```python
from build123d import *

# Parameters (mm, degrees)
SKETCH_R        = 2.25
SKETCH_R_2      = 11.25
SKETCH_R_3      = 1.75
PAD_DEPTH       = 23
POCKET_DEPTH    = 19
SKETCH003_R     = 4.05
POCKET002_DEPTH = 12


with BuildPart() as part:
    # Sketch → Pad (new body)
    with BuildSketch(Plane.XY):
        Polygon((0, 0), (105, 0), (105, 62), (20, 62), (20, 42), (0, 42), align=None)
        with Locations((35, 10)):
            Circle(SKETCH_R, mode=Mode.SUBTRACT)
        with Locations((30, 35)):
            Circle(SKETCH_R, mode=Mode.SUBTRACT)
        with Locations((84, 21)):
            Circle(SKETCH_R_2, mode=Mode.SUBTRACT)
        with Locations((68.5, 36.5)):
            Circle(SKETCH_R_3, mode=Mode.SUBTRACT)
        with Locations((99.5, 36.5)):
            Circle(SKETCH_R_3, mode=Mode.SUBTRACT)
        with Locations((68.5, 5.5)):
            Circle(SKETCH_R_3, mode=Mode.SUBTRACT)
        with Locations((99.5, 5.5)):
            Circle(SKETCH_R_3, mode=Mode.SUBTRACT)
        with Locations((10, 30)):
            Circle(SKETCH_R, mode=Mode.SUBTRACT)
        with Locations((10, 15)):
            Circle(SKETCH_R, mode=Mode.SUBTRACT)
        with Locations((39, 52)):
            Circle(SKETCH_R, mode=Mode.SUBTRACT)
        with Locations((94, 52)):
            Circle(SKETCH_R, mode=Mode.SUBTRACT)
        with Locations((55, 5)):
            Circle(SKETCH_R, mode=Mode.SUBTRACT)
        with BuildLine():
            Line((58.75, 25), (58.75, 40))
            ThreePointArc((58.75, 40), (56.5, 42.25), (54.25, 40))
            Line((54.25, 25), (54.25, 40))
            ThreePointArc((54.25, 25), (56.5, 22.75), (58.75, 25))
        make_face(mode=Mode.SUBTRACT)
    extrude(amount=PAD_DEPTH)

    # Sketch001 → Pocket (cut)
    with BuildSketch(Plane.XY.offset(23)):
        with BuildLine():
            ThreePointArc((38.485281, 42), (36.015595, 44.209377), (32.999996, 45.583006))
            Line((32.999996, 67), (32.999996, 45.583006))
            Line((20, 67), (32.999996, 67))
            Line((20, -1), (20, 67))
            Line((20, -1), (48.252269, -1))
            Line((48.252269, 11), (48.252269, -1))
            Line((48.252269, 11), (70.252269, 11))
            ThreePointArc((70.252269, 11), (71.759618, 9.202833), (73.499996, 7.630258))
            Line((73.499996, 7.630258), (73.499996, -1))
            Line((73.499996, -1), (93.499996, -1))
            Line((93.499996, -1), (93.499996, 6.902128))
            ThreePointArc((93.499996, 6.902128), (95.574295, 8.548671), (97.367695, 10.497399))
            Line((105.499996, 10.497399), (97.367695, 10.497399))
            Line((105.499996, 30.497399), (105.499996, 10.497399))
            Line((98.099621, 30.497399), (105.499996, 30.497399))
            ThreePointArc((98.099621, 30.497399), (91.98574, 36.007594), (83.999996, 38))
            Line((83.999996, 38), (83.999996, 67))
            Line((83.999996, 67), (43.999996, 67))
            Line((43.999996, 67), (43.999996, 42))
            Line((38.485281, 42), (43.999996, 42))
        make_face()
    extrude(amount=-POCKET_DEPTH, mode=Mode.SUBTRACT)

    # Sketch003 → Pocket002 (cut)
    with BuildSketch(Plane.XZ):
        with Locations((10, 16)):
            Circle(SKETCH003_R)
    extrude(amount=-POCKET002_DEPTH, mode=Mode.SUBTRACT)


solid = part.part
```
Geometry check sheet. Reference: the model listing, model coordinates, mm. A direction names the side the tool comes from. Give positions to 0.01 mm unless a question says otherwise; leave off trailing zeros. Write each loop counter-clockwise with the first axis right and the second up, starting at its lowest first coordinate (ties: lowest second). Pieces come first, ordered by that corner, then holes. Notation, with made-up numbers: (18.25, 35) -> (57.25, 35) arc R19 cw to (57.25, 45) -> close; hole circle Ø1 at (77, 23.5). An arc over 180 degrees is marked (long way). Use one line per item in the form item = value.
Item 1: Scan lines: line 1 (Y direction, x = 99.5, z = 12.5); line 2 (Y direction, x = 10, z = 13.25); line 3 (X direction, y = 32, z = 9). Record each from-to range of solid material in increasing order.
Results list:
line_1 = 0 to 3.75, 7.25 to 10.5, 30.5 to 34.75, 38.25 to 62
line_2 = 12 to 12.75, 17.25 to 27.75, 32.25 to 42
line_3 = 0 to 8.97, 11.03 to 20, 96.96 to 105
Item 2: Sectioned sample at C-C on y = 16. Enter the section's corners in (x, z).
Results list:
outline = (0, 0) -> (7.98, 0) -> (7.98, 23) -> (0, 23) -> close; (12.02, 0) -> (73.92, 0) -> (73.92, 4) -> (20, 4) -> (20, 23) -> (12.02, 23) -> close; (94.08, 0) -> (105, 0) -> (105, 4) -> (94.08, 4) -> close
Item 3: Mould release check, pull along Y, two halves, no side actions. Record for faces 1 (the flat face through (72.5, 62, 3.7)), 2 (the flat face through (93.5, 3, 14)), 3 (the cylindrical face through (99.12, 34.79, 11.34)): released by +Y, released by -Y, zero draft, split by the parting line, or undercut.
Results list:
face_1 = released by +Y
face_2 = zero draft
face_3 = undercut
Item 4: Sectioned sample at B-B on x = 99.5. Enter the section's corners in (y, z), plus the area to 3 significant figures.
Results list:
outline = (0, 0) -> (3.75, 0) -> (3.75, 23) -> (0, 23) -> close; (7.25, 0) -> (34.75, 0) -> (34.75, 23) -> (30.5, 23) -> (30.5, 4) -> (10.5, 4) -> (10.5, 23) -> (7.25, 23) -> close; (38.25, 0) -> (62, 0) -> (62, 23) -> (38.25, 23) -> close
area = 885 mm2
Item 5: Sectioned sample at A-A on z = 7.25. Count the separate pieces of the cut face and the enclosed holes in it, plus the area to 3 significant figures.
Results list:
separate_pieces = 5
enclosed_holes = 8
area = 1,910 mm2
Item 6: Access from +Z, -Z, +X, -X, +Y, -Y to the whole of each face (thin tool, end or side, straight path). Record for faces 4 (the flat face through (33, 54, 14)), 5 (the cylindrical face through (92, 36, 14)), 6 (the flat face through (44, 52, 14)).
Results list:
face_4 = +Z, -X, +Y, -Y
face_5 = +Z
face_6 = +Z, +Y, -Y
Item 7: Depth check by flat-ended pin: pin 1 Ø4 at (x, y) = (68.5, 36.5) entering from +Z; pin 2 Ø2 at (x, y) = (99.5, 5.5) entering from -Z; pin 3 Ø1 at (y, z) = (44.5, 7.5) entering from -X; pin 4 Ø4.5 at (y, z) = (50, 2) entering from -X. Enter the tip coordinate at first touch or a pass-through.
Results list:
pin_1 = 4
pin_2 = through
pin_3 = 34.58
pin_4 = 20
